from build123d import *

# Parameters (mm, degrees)
SKETCH1_W           = 95
SKETCH1_H           = 95
BOSS_EXTRUDE1_DEPTH = 1.6
SKETCH2_W           = 95
SKETCH2_H           = 95
SKETCH2_W_2         = 91.8
SKETCH2_H_2         = 91.8
BOSS_EXTRUDE2_DEPTH = 100
CUT_EXTRUDE1_DEPTH  = 147.982345879
FILLET1_R           = 5
SKETCH4_W           = 53
SKETCH4_H           = 22
CUT_EXTRUDE2_DEPTH  = 1.6
SKETCH5_R           = 1.65
CUT_EXTRUDE3_DEPTH  = 121.467838193
SKETCH6_W           = 60
SKETCH6_H           = 15
CUT_EXTRUDE4_DEPTH  = 1.6
FILLET2_R           = 5
BOSS_EXTRUDE3_START = 25
BOSS_EXTRUDE3_DEPTH = 2.4
CHAMFER1_SIZE       = 2.4


with BuildPart() as part:
    # Sketch1 → Boss-Extrude1 (new body)
    with BuildSketch(Plane(origin=(0, 0, 0), x_dir=(1, 0, 0), z_dir=(0, 1, 0))):
        Rectangle(SKETCH1_W, SKETCH1_H)
    extrude(amount=BOSS_EXTRUDE1_DEPTH)

    # Sketch2 → Boss-Extrude2 (add)
    with BuildSketch(Plane(origin=(0, 1.6, 0), x_dir=(1, 0, 0), z_dir=(0, 1, 0))):
        Rectangle(SKETCH2_W, SKETCH2_H)
        Rectangle(SKETCH2_W_2, SKETCH2_H_2, mode=Mode.SUBTRACT)
    extrude(amount=BOSS_EXTRUDE2_DEPTH)

    # Sketch3 → Cut-Extrude1 (cut, through all)
    with BuildSketch(Plane(origin=(47.5, 0, 0), x_dir=(0, 0, -1), z_dir=(1, 0, 0))):
        with BuildLine():
            Line((-47.5, 101.6), (47.5, 101.6))
            ThreePointArc((47.5, 101.6), (0, 96.6), (-47.5, 101.6))
        make_face()
    extrude(amount=-CUT_EXTRUDE1_DEPTH, mode=Mode.SUBTRACT)

    # Fillet1
    fillet1_edges = [part.edges().sort_by_distance(p)[0] for p in [
        (-45.9, 51.432685688, -45.9),
        (-45.9, 51.432685688, 45.9),
        (45.9, 51.432685688, -45.9),
        (45.9, 51.432685688, 45.9),
        (47.5, 50.8, 47.5),
        (-47.5, 50.8, 47.5),
        (-47.5, 50.8, -47.5),
        (47.5, 50.8, -47.5),
    ]]
    fillet(fillet1_edges, radius=FILLET1_R)

    # Sketch4 → Cut-Extrude2 (cut)
    with BuildSketch(Plane.ZY.offset(47.5)):
        with Locations((0, 11)):
            Rectangle(SKETCH4_W, SKETCH4_H)
    extrude(amount=-CUT_EXTRUDE2_DEPTH, mode=Mode.SUBTRACT)

    # Sketch5 → Cut-Extrude3 (cut, through all)
    with BuildSketch(Plane(origin=(0, 1.6, 0), x_dir=(1, 0, 0), z_dir=(0, 1, 0))):
        with Locations(Location((-22.4, 24.5, 0), (0, 0, 270))):
            Circle(SKETCH5_R)
        with Locations(Location((35.6, 24.5, 0), (0, 0, 270))):
            Circle(SKETCH5_R)
        with Locations(Location((35.6, -24.5, 0), (0, 0, 270))):
            Circle(SKETCH5_R)
        with Locations(Location((-22.4, -24.5, 0), (0, 0, 270))):
            Circle(SKETCH5_R)
    extrude(amount=-CUT_EXTRUDE3_DEPTH, mode=Mode.SUBTRACT)

    # Sketch6 → Cut-Extrude4 (cut)
    with BuildSketch(Plane(origin=(0, 0, -47.5), x_dir=(-1, 0, 0), z_dir=(0, 0, -1))):
        with Locations((-6.6, 7.5)):
            Rectangle(SKETCH6_W, SKETCH6_H)
    extrude(amount=-CUT_EXTRUDE4_DEPTH, mode=Mode.SUBTRACT)

    # Fillet2
    fillet2_edges = [part.edges().sort_by_distance(p)[0] for p in [
        (-23.4, 15, -46.7),
        (36.6, 15, -46.7),
    ]]
    fillet(fillet2_edges, radius=FILLET2_R)

    # Sketch7 → Boss-Extrude3 (add)
    with BuildSketch(Plane(origin=(0, 1.6, 0), x_dir=(1, 0, 0), z_dir=(0, 1, 0)).offset(BOSS_EXTRUDE3_START)):
        with BuildLine():
            Line((-40.9, -45.9), (40.9, -45.9))
            ThreePointArc((40.9, -45.9), (44.435533906, -44.435533906), (45.9, -40.9))
            Line((45.9, -40.9), (45.9, 40.9))
            ThreePointArc((45.9, 40.9), (44.435533906, 44.435533906), (40.9, 45.9))
            Line((40.9, 45.9), (36.6, 45.9))
            Line((36.6, 45.9), (-23.4, 45.9))
            Line((-23.4, 45.9), (-40.9, 45.9))
            ThreePointArc((-40.9, 45.9), (-44.435533906, 44.435533906), (-45.9, 40.9))
            Line((-45.9, 40.9), (-45.9, 26.5))
            Line((-45.9, 26.5), (-45.9, -26.5))
            Line((-45.9, -26.5), (-45.9, -40.9))
            ThreePointArc((-45.9, -40.9), (-44.435533906, -44.435533906), (-40.9, -45.9))
        make_face()
        with BuildLine():
            Line((-40.9, -43.5), (40.9, -43.5))
            ThreePointArc((40.9, -43.5), (42.738477631, -42.738477631), (43.5, -40.9))
            Line((43.5, -40.9), (43.5, 40.9))
            ThreePointArc((43.5, 40.9), (42.738477631, 42.738477631), (40.9, 43.5))
            Line((40.9, 43.5), (36.6, 43.5))
            Line((36.6, 43.5), (-23.4, 43.5))
            Line((-23.4, 43.5), (-40.9, 43.5))
            ThreePointArc((-40.9, 43.5), (-42.738477631, 42.738477631), (-43.5, 40.9))
            Line((-43.5, 40.9), (-43.5, 26.5))
            Line((-43.5, 26.5), (-43.5, -26.5))
            Line((-43.5, -26.5), (-43.5, -40.9))
            ThreePointArc((-43.5, -40.9), (-42.738477631, -42.738477631), (-40.9, -43.5))
        make_face(mode=Mode.SUBTRACT)
    extrude(amount=-BOSS_EXTRUDE3_DEPTH)

    # Chamfer1
    chamfer1_edges = [part.edges().sort_by_distance(p)[0] for p in [
        (0, 24.2, 43.5),
        (42.738477631, 24.2, 42.738477631),
        (-42.738477631, 24.2, 42.738477631),
        (43.5, 24.2, 0),
        (-43.5, 24.2, 0),
        (42.738477631, 24.2, -42.738477631),
        (-42.738477631, 24.2, -42.738477631),
        (0, 24.2, -43.5),
    ]]
    chamfer(chamfer1_edges, length=CHAMFER1_SIZE - 0.0001)  # a hair under: the kernel refuses the full size


solid = part.part
Part model, mm, in its own coordinate system. A direction names the side the tool comes from. Coordinates: 2 decimals unless noted, no trailing zeros. Order: outer loops, then holes, each group sorted by start corner. A loop starts at its lowest first (then second) coordinate and runs counter-clockwise, first axis right, second up. Notation, with made-up numbers: M -13.75,39.5 L 21.25,39.5 A36 ccw 21.25,75.5 Z; hole C 19.25,-33 d11. An arc over 180 degrees is marked long. Use a Markdown table: item, result.
(1) Pull direction Z, two halves, no side cores. Call faces 4 (the flat face through (45.9, 13, 1)), 5 (the cylindrical face through (46, 51.51, 46.07)), 6 (the cylindrical face through (46, 50.09, -46.07)): released by +Z, released by -Z, zero draft, split by the parting line, or undercut.
A:
| item | result |
|---|---|
| face 4 | undercut |
| face 5 | released by +Z |
| face 6 | released by -Z |
(2) Cut at A-A on y = 63. Write the cut outline in (x, z).
A:
| item | result |
|---|---|
| outline | M -47.5,-42.5 A5 ccw -42.5,-47.5 L 42.5,-47.5 A5 ccw 47.5,-42.5 L 47.5,42.5 A5 ccw 42.5,47.5 L -42.5,47.5 A5 ccw -47.5,42.5 Z; hole M -45.9,-40.9 A5 ccw -40.9,-45.9 L 40.9,-45.9 A5 ccw 45.9,-40.9 L 45.9,40.9 A5 ccw 40.9,45.9 L -40.9,45.9 A5 ccw -45.9,40.9 Z |
(3) Tool access for faces 1 (the cylindrical face through (-46.07, 51.51, 46)), 2 (the conical face through (-43.414, 25.683, 43.359)), 3 (the flat face through (-1, 63, 45.9)): list every direction of +Z, -Z, +X, -X, +Y, -Y with a clear straight run to the whole face (end or side of a thin tool).
A:
| item | result |
|---|---|
| face 1 | +Z, -X, +Y, -Y |
| face 2 | none |
| face 3 | +Y |
(4) Flat gauge pins, fed straight in: pin 1 (1.3 mm diameter, centred on y = 5.5, z = -46.5, fed in from +X); pin 2 (0.5 mm diameter, centred on x = -47, z = -3, fed in from -Y); pin 3 (0.5 mm diameter, centred on x = -47, y = 16.5, fed in from -Z); pin 4 (2.5 mm diameter, centred on x = 35.6, z = -24.5, fed in from +Y). Where does each tip first touch, or does it go through?
A:
| item | result |
|---|---|
| pin 1 | stops at x = 46.21 |
| pin 2 | stops at y = 22 |
| pin 3 | stops at z = -45.13 |
| pin 4 | passes through |
(5) Probe L1, parallel to X at y = 0.45, z = -24.5; L2, parallel to Z at x = -24.5, y = 45. List the from-to ranges inside material, lowest first.
A:
| item | result |
|---|---|
| L1 | x = -45.9 to -24.05, -20.75 to 33.95, 37.25 to 47.5 |
| L2 | z = -47.5 to -45.9, 45.9 to 47.5 |
